Build history of the part. All positions in model axes, mm. A direction names the side the tool comes from. Round coordinates to 2 decimals unless told otherwise and drop trailing zeros. Write each loop counter-clockwise with the first axis right and the second up, starting at its lowest first coordinate (ties: lowest second). Pieces come first, ordered by that corner, then holes. Notation, with made-up numbers: M 38.25,-13 L 77.25,-13 A15 ccw 77.25,-2 Z; hole C 43.25,18.5 d2. An arc over 180 degrees is marked long. Use a Markdown table: item, result.
from build123d import *

# Parameters (mm, degrees)
SKETCH1_W                  = 109.5
SKETCH1_H                  = 82.5
BOSS_EXTRUDE1_DEPTH        = 2
F_3_5_3_5_DIAMETER_HOLE1_D = 3.5
F_2_5_2_5_DIAMETER_HOLE1_D = 2.5
F_2_6_2_6_DIAMETER_HOLE1_D = 2.6
SKETCH9_R                  = 3
CUT_EXTRUDE1_DEPTH         = 1
F_2_2_2_2_DIAMETER_HOLE1_D = 2.2
FILLET1_R                  = 1
FILLET2_R                  = 3


with BuildPart() as part:
    # Sketch1 → Boss-Extrude1 (new body)
    with BuildSketch(Plane.XY):
        with Locations((0, -41.75)):
            Rectangle(SKETCH1_W, SKETCH1_H)
        with BuildLine():
            Line((28.75, -9.25), (28.75, -13.6))
            ThreePointArc((28.75, -13.6), (29.628679656, -15.721320344), (31.75, -16.6))
            Line((31.75, -16.6), (41.75, -16.6))
            ThreePointArc((41.75, -16.6), (43.871320344, -17.478679656), (44.75, -19.6))
            Line((44.75, -19.6), (44.75, -31.75))
            Line((44.75, -31.75), (48.75, -31.75))
            Line((48.75, -31.75), (48.75, -41.75))
            Line((48.75, -41.75), (48.75, -51.75))
            Line((48.75, -51.75), (44.75, -51.75))
            Line((44.75, -51.75), (44.75, -74.25))
            ThreePointArc((44.75, -74.25), (43.871320344, -76.371320344), (41.75, -77.25))
            Line((41.75, -77.25), (-41.75, -77.25))
            ThreePointArc((-41.75, -77.25), (-43.871320344, -76.371320344), (-44.75, -74.25))
            Line((-44.75, -74.25), (-44.75, -51.75))
            Line((-44.75, -51.75), (-48.75, -51.75))
            Line((-48.75, -51.75), (-48.75, -31.75))
            Line((-48.75, -31.75), (-44.75, -31.75))
            Line((-44.75, -31.75), (-44.75, -9.25))
            ThreePointArc((-44.75, -9.25), (-43.871320344, -7.128679656), (-41.75, -6.25))
            Line((-41.75, -6.25), (25.75, -6.25))
            ThreePointArc((25.75, -6.25), (27.871320344, -7.128679656), (28.75, -9.25))
        make_face(mode=Mode.SUBTRACT)
    extrude(amount=BOSS_EXTRUDE1_DEPTH)

    # Ø3.5 (3.5) Diameter Hole1 (through all)
    with Locations(Plane.XY.offset(2)):
        with Locations((-48.25, -3.75), (-48.25, -79.75), (48.25, -79.75), (48.25, -3.75)):
            Hole(F_3_5_3_5_DIAMETER_HOLE1_D / 2)

    # Ø2.5 (2.5) Diameter Hole1 (through all)
    with Locations(Plane.XY.offset(2)):
        with Locations((33.65, -12.1)):
            Hole(F_2_5_2_5_DIAMETER_HOLE1_D / 2)

    # Ø2.6 (2.6) Diameter Hole1 (through all)
    with Locations(Plane.XY.offset(2)):
        with Locations((33.65, -2.57)):
            Hole(F_2_6_2_6_DIAMETER_HOLE1_D / 2)

    # Sketch9 → Cut-Extrude1 (cut)
    with BuildSketch(Plane.XY.offset(2)):
        with Locations((-48.25, -3.75)):
            Circle(SKETCH9_R)
        with Locations((48.25, -3.75)):
            Circle(SKETCH9_R)
        with Locations((48.25, -79.75)):
            Circle(SKETCH9_R)
        with Locations((-48.25, -79.75)):
            Circle(SKETCH9_R)
    extrude(amount=-CUT_EXTRUDE1_DEPTH, mode=Mode.SUBTRACT)

    # Ø2.2 (2.2) Diameter Hole1 (through all)
    with Locations(Plane.XY.offset(2)):
        with Locations((-24.75, -3.25), (24.75, -3.25), (-24.75, -80.25), (24.75, -80.25)):
            Hole(F_2_2_2_2_DIAMETER_HOLE1_D / 2)

    # Fillet1
    fillet1_edges = [part.edges().sort_by_distance(p)[0] for p in [
        (-44.75, -31.75, 1),
        (-44.75, -51.75, 1),
        (44.75, -51.75, 1),
        (44.75, -31.75, 1),
    ]]
    fillet(fillet1_edges, radius=FILLET1_R)

    # Fillet2
    fillet2_edges = [part.edges().sort_by_distance(p)[0] for p in [
        (48.75, -31.75, 1),
        (48.75, -51.75, 1),
        (-48.75, -51.75, 1),
        (-48.75, -31.75, 1),
    ]]
    fillet(fillet2_edges, radius=FILLET2_R - 0.0001)  # a hair under: the kernel refuses the full size


solid = part.part
Q1. Cut at A-A on y = -71. Give the cut face in (x, z).
Response values:
| item | result |
|---|---|
| outline | M -54.75,0 L -44.75,0 L -44.75,2 L -54.75,2 Z; M 44.75,0 L 54.75,0 L 54.75,2 L 44.75,2 Z |
Q2. Two-plate mould, pull along Y, no slides. Class faces 1 (the flat face through (50, -81, 1)), 2 (the flat face through (-8, -5, 2)): +Y half, -Y half, draft (parallel to the pull), parting line (faces both ways), or undercut.
Response values:
| item | result |
|---|---|
| face 1 | undercut |
| face 2 | draft |
Q3. Cut at B-B on x = 15. Give the cut face in (y, z), and give its area (3 significant figures).
Response values:
| item | result |
|---|---|
| outline | M -83,0 L -77.25,0 L -77.25,2 L -83,2 Z; M -6.25,0 L -0.5,0 L -0.5,2 L -6.25,2 Z |
| area | 23.0 mm2 |
Q4. Drop flat-ended pins along their axis: P1, Ø2, axis at x = -48.25, y = -3.75, coming from the -Z side; P2, Ø3.5, axis at x = 33.65, y = -2.57, coming from the +Z side; P3, Ø4.5, axis at x = 48.25, y = -3.75, coming from the +Z side. Give the stop position or say it passes through.
Response values:
| item | result |
|---|---|
| P1 | passes through |
| P2 | stops at z = 2 |
| P3 | stops at z = 1 |
Q5. Cut at D-D on z = 0.55. Count the separate pieces of the cut face and the enclosed holes in it, and give its area (3 significant figures).
Response values:
| item | result |
|---|---|
| separate pieces | 1 |
| enclosed holes | 11 |
| area | 2,640 mm2 |
Q6. Which spindle directions (+Z, -Z, +X, -X, +Y, -Y) get a long thin tool onto all of the face, cutting with end or side? Do faces 3 (the cylindrical face through (45.253, -3.618, 1.507)), 4 (the flat face through (-8, -5, 0)), 5 (the cylindrical face through (29.61, -15.7, 0.99)). Say none if no direction does.
Response values:
| item | result |
|---|---|
| face 3 | +Z |
| face 4 | -Z, +X, -X, +Y, -Y |
| face 5 | +Z, -Z |
Q7. Cut at C-C on x = 33.65. Give the cut face in (y, z).
Response values:
| item | result |
|---|---|
| outline | M -83,0 L -77.25,0 L -77.25,2 L -83,2 Z; M -16.6,0 L -13.35,0 L -13.35,2 L -16.6,2 Z; M -10.85,0 L -3.87,0 L -3.87,2 L -10.85,2 Z; M -1.27,0 L -0.5,0 L -0.5,2 L -1.27,2 Z |
Q8. Drill centre lines: L1, parallel to Y at x = 33.65, z = 1.45; L2, parallel to Y at x = -9, z = 0.75; L3, parallel to X at y = -63.5, z = 0.65. Where is each one in solid material? Low to high.
Response values:
| item | result |
|---|---|
| L1 | y = -83 to -77.25, -16.6 to -13.35, -10.85 to -3.87, -1.27 to -0.5 |
| L2 | y = -83 to -77.25, -6.25 to -0.5 |
| L3 | x = -54.75 to -44.75, 44.75 to 54.75 |
